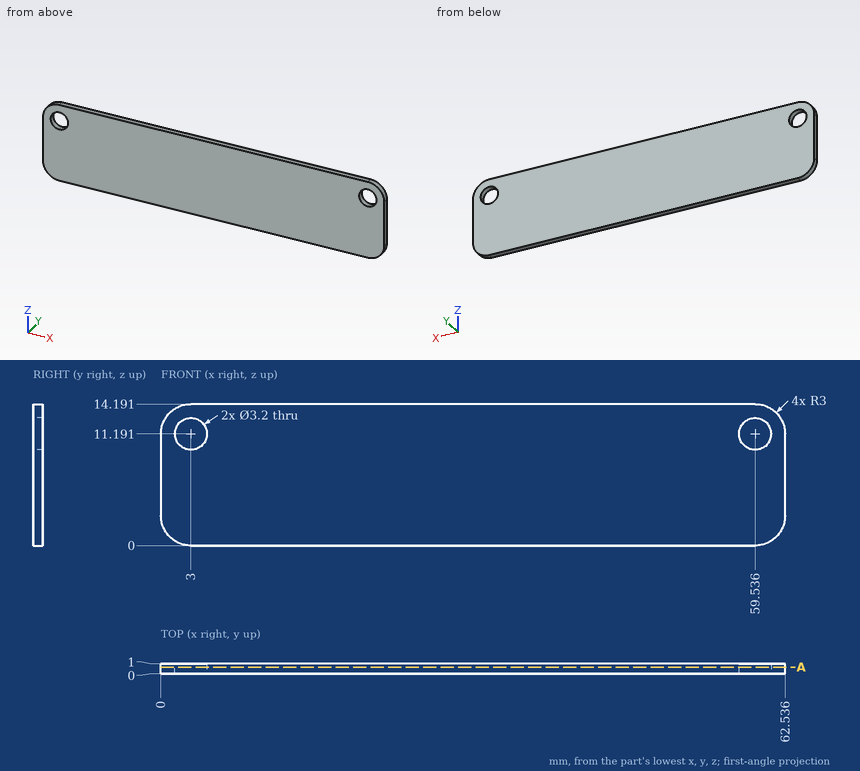
Geometry check sheet. Reference: drawing and pictorial views, mm from the part's lowest x, y, z. Round coordinates to 2 decimals unless told otherwise and drop trailing zeros. Order: outer loops, then holes, each group sorted by start corner. A loop starts at its lowest first (then second) coordinate and runs counter-clockwise, first axis right, second up. Notation, with made-up numbers: (68.25, -18.5) - (107.25, -18.5) arc R16 cw to (107.25, -3.5) - close; hole circle Ø11 at (20.5, 19). An arc over 180 degrees is marked (long way). Use a Markdown table: item, result. Add a question column.
1) Section check A-A (y = 0.65). Record the cut outline in (x, z) (1 decimal), then the cut area to 3 significant figures.
2) Gauge pin test, flat ends, axial feed: P1, Ø3, axis at x = 3, z = 11.19, coming from the -Y side; P2, Ø4, axis at x = 59.54, z = 11.19, coming from the +Y side. Record the tip position at first contact, or that the pin passes through.
3) Thickness scan on line 1 along X through (y, z) = (0.4, 11.5) (1 decimal); line 2 along Z through (x, y) = (3, 0.55); line 3 along X through (y, z) = (0.5, 12) (1 decimal). Record the ranges inside material, lowest first.
Established:
| question | item | result |
|---|---|---|
| 1 | outline | (0, 3) arc R3 ccw to (3, 0) - (59.5, 0) arc R3 ccw to (62.5, 3) - (62.5, 11.2) arc R3 ccw to (59.5, 14.2) - (3, 14.2) arc R3 ccw to (0, 11.2) - close; hole circle Ø3.2 at (3, 11.2); hole circle Ø3.2 at (59.5, 11.2) |
| 1 | area | 864 mm2 |
| 2 | P1 | through |
| 2 | P2 | y = 1 |
| 3 | line 1 | 0 to 1.4, 4.6 to 58, 61.1 to 62.5 |
| 3 | line 2 | 0 to 9.59, 12.79 to 14.19 |
| 3 | line 3 | 0.1 to 1.6, 4.4 to 58.2, 60.9 to 62.4 |
